For this review, use the dimensioned drawing (mm, ordinates from the lowest corner) and the shaded views. A direction names the side the tool comes from. Coordinates: 2 decimals unless noted, no trailing zeros. Write each loop counter-clockwise with the first axis right and the second up, starting at its lowest first coordinate (ties: lowest second). Pieces come first, ordered by that corner, then holes. Notation, with made-up numbers: M 23.5,9 L 54.5,9 A16 cw 54.5,13 Z; hole C 31,55.5 d6. An arc over 180 degrees is marked long. One line per question, with ' | ' between items.
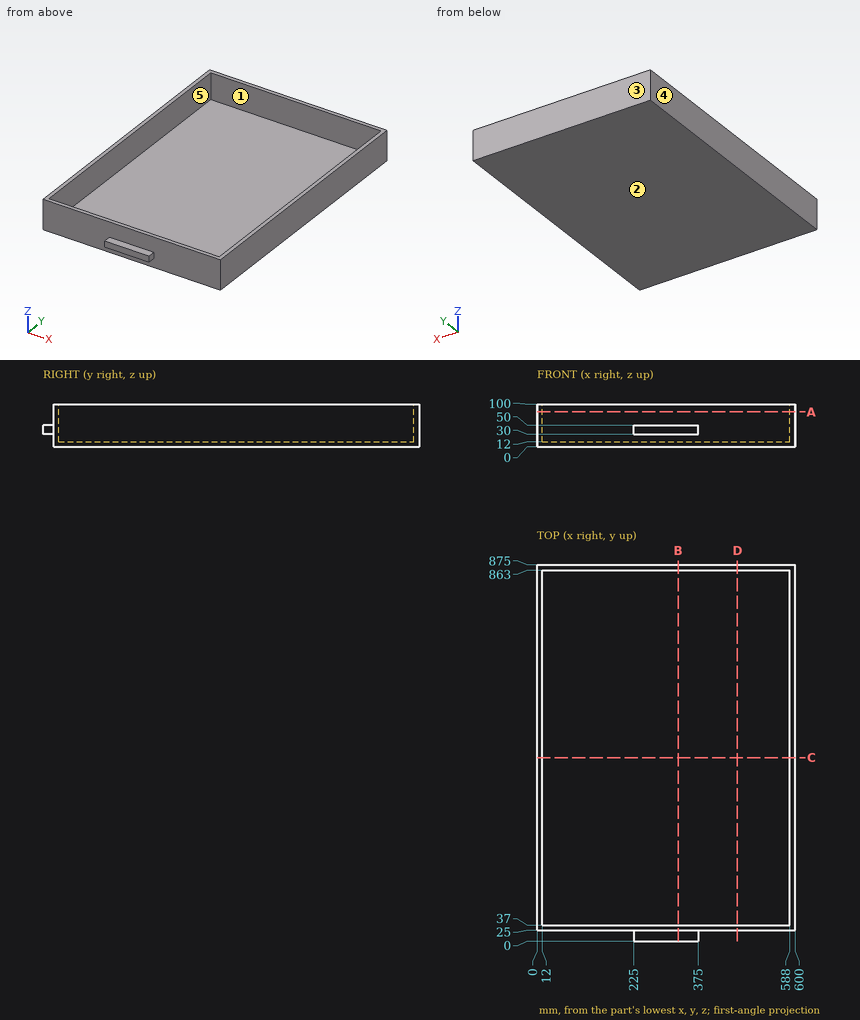
1) The part is to be moulded in two halves that separate along Y. For the marked faces 3, 4 and 5, say which applies: +Y half, -Y half, draft (parallel to the pull), parting line (faces both ways), or undercut.
Responses:
face 3: +Y half | face 4: draft | face 5: undercut
2) Machinability: for the marked faces 1 and 2, which of the approach directions +Z, -Z, +X, -X, +Y, -Y give a long, thin tool a straight path to every point of the face, cutting with its end or side? Answer none if there is none.
Responses:
face 1: +Z | face 2: -Z, +X, -X, +Y, -Y
3) We need section B-B on x = 328. State the section outline as (y, z) points, then the cut area to 3 significant figures.
Responses:
outline: M 0,30 L 25,30 L 25,0 L 875,0 L 875,100 L 863,100 L 863,12 L 37,12 L 37,100 L 25,100 L 25,50 L 0,50 Z | area: 12,800 mm^2
4) We need section A-A on z = 81.5. State the section outline as (x, y) points, then the cut area to 3 significant figures.
Responses:
outline: M 0,25 L 600,25 L 600,875 L 0,875 Z; hole M 12,37 L 588,37 L 588,863 L 12,863 Z | area: 34,200 mm^2
5) To check wall thickness, follow line 1 along X through (y, z) = (183.5, 40.5); line 2 along Y through (x, z) = (222.5, 54.5); line 3 along Z through (x, y) = (181.5, 574). State the ranges of each line that lie inside material, in increasing order. Write a range as [from, to].
Responses:
line 1: [0, 12], [588, 600] | line 2: [25, 37], [863, 875] | line 3: [0, 12]
6) We need section D-D on x = 466. State the section outline as (y, z) points.
Responses:
outline: M 25,0 L 875,0 L 875,100 L 863,100 L 863,12 L 37,12 L 37,100 L 25,100 Z
7) Insertion check: pin 1 Ø1.5 at (x, z) = (325, 10.5) entering from -Y; pin 2 Ø1 at (x, y) = (374, 212.5) entering from +Z; pin 3 Ø22 at (y, z) = (13, 40.5) entering from -X. Each pin has a flat end and moves straight along its axis. Give the tip position at first contact, or say it passes through.
Responses:
pin 1: y = 25 | pin 2: z = 12 | pin 3: x = 225
8) We need section C-C on y = 427. State the section outline as (x, z) points.
Responses:
outline: M 0,0 L 600,0 L 600,100 L 588,100 L 588,12 L 12,12 L 12,100 L 0,100 Z
